Part print with two shaded views. Sizes in mm from the minimum x, y, z corner. A direction names the side the tool comes from. Round coordinates to 2 decimals unless told otherwise and drop trailing zeros. Loops run counter-clockwise (first coordinate to the right, second up) from the corner with the lowest first, then second, coordinate; pieces in that order, holes last.
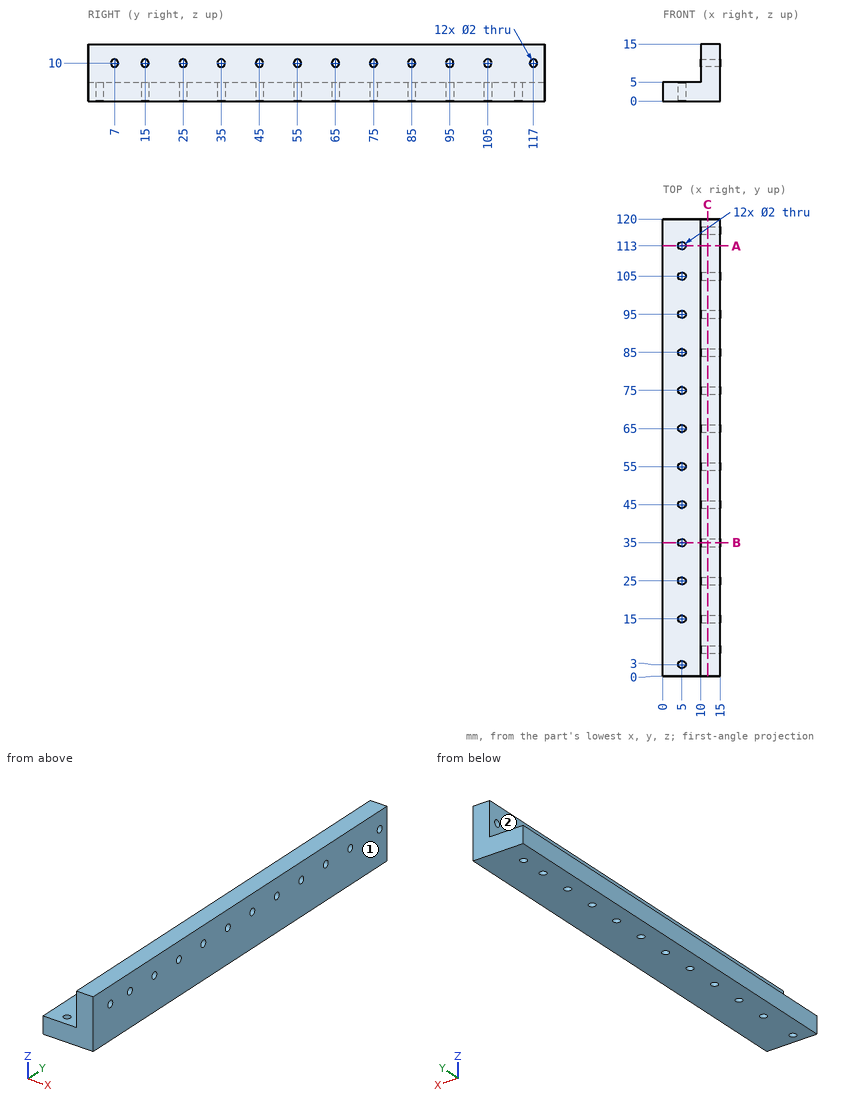
Item 1: Wall check: L1, parallel to Z at x = 6.75, y = 12.5; L2, parallel to X at y = 65, z = 1; L3, parallel to X at y = 47.5, z = 8.5. Give the ranges that are in metal, low to high.
Verdict:
L1: z = 0 to 5
L2: x = 0 to 4, 6 to 15
L3: x = 10 to 15
Item 2: 3-axis set-ups, long thin cutter, end or side, ignore diameter. For the marked faces 1 and 2: which of +Z, -Z, +X, -X, +Y, -Y reach the whole face in a straight line?
Verdict:
face 1: +Z, -Z, +X, +Y, -Y
face 2: +Z, -X, +Y, -Y
Item 3: Cut at A-A (y = 113). List the corners of the cut face in (x, z), plus the area to 3 significant figures.
Verdict:
outline: (0, 0) - (4, 0) - (4, 5) - (0, 5) - close; (6, 0) - (15, 0) - (15, 15) - (10, 15) - (10, 5) - (6, 5) - close
area: 115 mm2
Item 4: Cut at B-B (y = 35). List the corners of the cut face in (x, z).
Verdict:
outline: (0, 0) - (4, 0) - (4, 5) - (0, 5) - close; (6, 0) - (15, 0) - (15, 9) - (10, 9) - (10, 5) - (6, 5) - close; (10, 11) - (15, 11) - (15, 15) - (10, 15) - close
Item 5: Cut at C-C (x = 11.75). State how many separate pieces and enclosed holes the cut face has, plus the area to 3 significant figures.
Verdict:
separate pieces: 1
enclosed holes: 12
area: 1,760 mm2
Item 6: Flat gauge pins, fed straight in: P1, Ø1.5, axis at x = 12.5, y = 71, coming from the -Z side; P2, Ø1, axis at y = 14.5, z = 10.5, coming from the -X side; P3, Ø1.8, axis at x = 5, y = 95, coming from the -Z side; P4, Ø3, axis at x = 5, y = 25, coming from the +Z side. Where does each tip first touch, or does it go through?
Verdict:
P1: stops at z = 0
P2: stops at x = 10
P3: passes through
P4: stops at z = 5
